Check sheet for the modelled part. Datum: model origin and axes. Units: mm. Round coordinates to 2 decimals unless told otherwise and drop trailing zeros. Loops run counter-clockwise (first coordinate to the right, second up) from the corner with the lowest first, then second, coordinate; pieces in that order, holes last. Notation, with made-up numbers: (71, -17) -> (95, -17) arc R16 ccw to (95, 9) -> close; hole circle Ø9 at (-5.75, 18). An arc over 180 degrees is marked (long way). Use one line per item in the form item = value. Start each with the question number.
(1) Sectioned sample at A-A (z = 0). Record the cut outline in (x, y).
(2) Sectioned sample at B-B (x = 179). Record the cut outline in (y, z).
(3) Go/stop test with flat-tipped pins: pin 1 (12 mm diameter, centred on y = 5.5, z = -6.5, fed in from +X); pin 2 (5 mm diameter, centred on y = -6.5, z = 8, fed in from +X); pin 3 (3 mm diameter, centred on x = 74.5, z = 3.5, fed in from -Y); pin 4 (2 mm diameter, centred on x = 37.5, y = -1, fed in from -Z). Record where each tip stops, or that it passes through.
(4) Sectioned sample at D-D (z = 14). Record the cut outline in (x, y), and give its area (3 significant figures).
(5) Material ranges on probe 1 along X at (y, z) = (6, 13); probe 2 along Z at (x, y) = (338, 1.5); probe 3 along Z at (x, y) = (168.5, 0.5), recorded low to high. Write a range as [from, to].
(6) Sectioned sample at C-C (y = -13.5). Record the cut outline in (x, z), and give its area (3 significant figures).
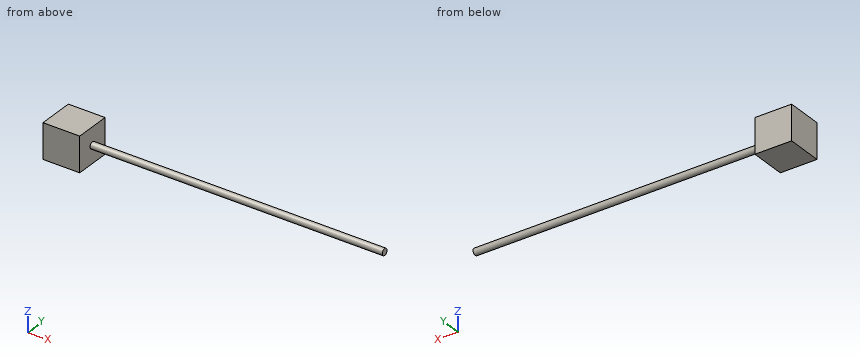
from build123d import *

# Parameters (mm, degrees)
CROQUIS1_W              = 44
CROQUIS1_H              = 42
SALIENTE_EXTRUIR1_DEPTH = 21.5
CROQUIS2_R              = 4
SALIENTE_EXTRUIR2_DEPTH = 350


with BuildPart() as part:
    # Croquis1 → Saliente-Extruir1 (new, symmetric)
    with BuildSketch(Plane(origin=(0, 0, 0), x_dir=(1, 0, 0), z_dir=(0, 1, 0))):
        Rectangle(CROQUIS1_W, CROQUIS1_H)
    extrude(amount=SALIENTE_EXTRUIR1_DEPTH, both=True)

    # Croquis2 → Saliente-Extruir2 (add)
    with BuildSketch(Plane(origin=(22, 0, 0), x_dir=(0, 0, -1), z_dir=(1, 0, 0))):
        with Locations(Location((0, 0, 0), (0, 0, 180))):
            Circle(CROQUIS2_R)
    extrude(amount=SALIENTE_EXTRUIR2_DEPTH)


solid = part.part
Checks:
q1.outline = (-22, -21.5) -> (22, -21.5) -> (22, -4) -> (372, -4) -> (372, 4) -> (22, 4) -> (22, 21.5) -> (-22, 21.5) -> close
q2.outline = circle Ø8 at (0, 0)
q3.pin_1 = 372
q3.pin_2 = 22
q3.pin_3 = -3.46
q3.pin_4 = -4
q4.outline = (-22, -21.5) -> (22, -21.5) -> (22, 21.5) -> (-22, 21.5) -> close
q4.area = 1,890 mm2
q5.probe_1 = [-22, 22]
q5.probe_2 = [-3.71, 3.71]
q5.probe_3 = [-3.97, 3.97]
q6.outline = (-22, -21) -> (22, -21) -> (22, 21) -> (-22, 21) -> close
q6.area = 1,850 mm2
